Source: CAD feature listing. Evaluate the final solid. Frame: model axes, mm. Face numbers are marked on the shaded views. Give positions to 0.01 mm unless a question says otherwise; leave off trailing zeros. Order: outer loops, then holes, each group sorted by start corner. A loop starts at its lowest first (then second) coordinate and runs counter-clockwise, first axis right, second up. Notation, with made-up numbers: (-37, -14.5) -> (7, -14.5) arc R31 cw to (7, 10.5) -> close; hole circle Ø3 at (81.25, 16). An arc over 180 degrees is marked (long way). Answer in a Markdown table with one row per item.
Autodesk Inventor part; units mm, degrees
ref_plane "mss_or_XY" through (0, 0, 0) normal (1, 0, 0) x (0, 0, -1)
ref_plane "mss_or_YZ" through (0, 0, 0) normal (0, 0, -1) x (0, 1, 0)
ref_plane "mss_or_ZX" through (0, 0, 0) normal (0, 1, 0) x (1, 0, 0)
sketch "Sketch_2" plane through (0, 0, 0) normal (0, 0, 1) x (1, 0, 0)
  line L0 (2.5, 0) -> (0, 0)
  line L1 (0, 2.92) -> (0, 2.52)
  line L2 (0, 2.52) -> (0.8975, 2.52)
  arc A0 (1.6025, 2.52) -> (0.8975, 2.52) centre (1.25, 2.25) ccw
  line L3 (1.6025, 2.52) -> (2.4438, 2.52)
  line L4 (2.4438, 2.52) -> (2.4438, 2.616)
  line L5 (2.4438, 2.616) -> (2.5, 2.616)
  line L6 (2.5, 2.616) -> (2.5, 2.92)
  arc A1 (2.5, 2.92) -> (2.42, 3) centre (2.42, 2.92) ccw
  line L7 (2.42, 3) -> (0.08, 3)
  arc A2 (0.08, 3) -> (0, 2.92) centre (0.08, 2.92) ccw
revolve "Revolution1" add sketch "Sketch_2" angle 360 about axis through (2.5, 0, 0) along (1, 0, 0)
ref_plane "mss_or_XY" through (0, 0, 0) normal (1, 0, 0) x (0, 0, -1)
ref_plane "mss_or_YZ" through (0, 0, 0) normal (0, 0, -1) x (0, 1, 0)
ref_plane "mss_or_ZX" through (0, 0, 0) normal (0, 1, 0) x (1, 0, 0)
ref_plane "mss_or11_XY" through (2.5, 0, 0) normal (1, 0, 0) x (0, 0, -1)
ref_plane "mss_or11_YZ" through (2.5, 0, 0) normal (0, 0, -1) x (0, 1, 0)
ref_plane "mss_or11_ZX" through (2.5, 0, 0) normal (0, 1, 0) x (1, 0, 0)
ref_plane "mss_or2_1_XY" through (1, 2.25, 0) normal (1, 0, 0) x (0, 0, -1)
ref_plane "mss_or2_1_YZ" through (1, 2.25, 0) normal (0, 0, -1) x (0, 1, 0)
ref_plane "mss_or2_1_ZX" through (1, 2.25, 0) normal (0, 1, 0) x (1, 0, 0)
ref_plane "mss_or2_2_XY" through (1, 1.7236, 1.4463) normal (1, 0, 0) x (0, 0, -1)
ref_plane "mss_or2_2_YZ" through (1, 1.7236, 1.4463) normal (0, 0, -1) x (0, 1, 0)
ref_plane "mss_or2_2_ZX" through (1, 1.7236, 1.4463) normal (0, 1, 0) x (1, 0, 0)
ref_plane "mss_or2_3_XY" through (1, 0.3907, 2.2158) normal (1, 0, 0) x (0, 0, -1)
ref_plane "mss_or2_3_YZ" through (1, 0.3907, 2.2158) normal (0, 0, -1) x (0, 1, 0)
ref_plane "mss_or2_3_ZX" through (1, 0.3907, 2.2158) normal (0, 1, 0) x (1, 0, 0)
ref_plane "mss_or2_4_XY" through (1, -1.125, 1.9486) normal (1, 0, 0) x (0, 0, -1)
ref_plane "mss_or2_4_YZ" through (1, -1.125, 1.9486) normal (0, 0, -1) x (0, 1, 0)
ref_plane "mss_or2_4_ZX" through (1, -1.125, 1.9486) normal (0, 1, 0) x (1, 0, 0)
ref_plane "mss_or2_5_XY" through (1, -2.1143, 0.7695) normal (1, 0, 0) x (0, 0, -1)
ref_plane "mss_or2_5_YZ" through (1, -2.1143, 0.7695) normal (0, 0, -1) x (0, 1, 0)
ref_plane "mss_or2_5_ZX" through (1, -2.1143, 0.7695) normal (0, 1, 0) x (1, 0, 0)
ref_plane "mss_or2_6_XY" through (1, -2.1143, -0.7695) normal (1, 0, 0) x (0, 0, -1)
ref_plane "mss_or2_6_YZ" through (1, -2.1143, -0.7695) normal (0, 0, -1) x (0, 1, 0)
ref_plane "mss_or2_6_ZX" through (1, -2.1143, -0.7695) normal (0, 1, 0) x (1, 0, 0)
ref_plane "mss_or2_7_XY" through (1, -1.125, -1.9486) normal (1, 0, 0) x (0, 0, -1)
ref_plane "mss_or2_7_YZ" through (1, -1.125, -1.9486) normal (0, 0, -1) x (0, 1, 0)
ref_plane "mss_or2_7_ZX" through (1, -1.125, -1.9486) normal (0, 1, 0) x (1, 0, 0)
ref_plane "mss_or2_8_XY" through (1, 0.3907, -2.2158) normal (1, 0, 0) x (0, 0, -1)
ref_plane "mss_or2_8_YZ" through (1, 0.3907, -2.2158) normal (0, 0, -1) x (0, 1, 0)
ref_plane "mss_or2_8_ZX" through (1, 0.3907, -2.2158) normal (0, 1, 0) x (1, 0, 0)
ref_plane "mss_or2_9_XY" through (1, 1.7236, -1.4463) normal (1, 0, 0) x (0, 0, -1)
ref_plane "mss_or2_9_YZ" through (1, 1.7236, -1.4463) normal (0, 0, -1) x (0, 1, 0)
ref_plane "mss_or2_9_ZX" through (1, 1.7236, -1.4463) normal (0, 1, 0) x (1, 0, 0)
ref_plane "mss_or21_1_XY" through (1.25, 2.25, 0) normal (1, 0, 0) x (0, 0, -1)
ref_plane "mss_or21_1_YZ" through (1.25, 2.25, 0) normal (0, 0, -1) x (0, 1, 0)
ref_plane "mss_or21_1_ZX" through (1.25, 2.25, 0) normal (0, 1, 0) x (1, 0, 0)
ref_plane "mss_or21_2_XY" through (1.25, 1.7236, 1.4463) normal (1, 0, 0) x (0, 0, -1)
ref_plane "mss_or21_2_YZ" through (1.25, 1.7236, 1.4463) normal (0, 0, -1) x (0, 1, 0)
ref_plane "mss_or21_2_ZX" through (1.25, 1.7236, 1.4463) normal (0, 1, 0) x (1, 0, 0)
ref_plane "mss_or21_3_XY" through (1.25, 0.3907, 2.2158) normal (1, 0, 0) x (0, 0, -1)
ref_plane "mss_or21_3_YZ" through (1.25, 0.3907, 2.2158) normal (0, 0, -1) x (0, 1, 0)
ref_plane "mss_or21_3_ZX" through (1.25, 0.3907, 2.2158) normal (0, 1, 0) x (1, 0, 0)
ref_plane "mss_or21_4_XY" through (1.25, -1.125, 1.9486) normal (1, 0, 0) x (0, 0, -1)
ref_plane "mss_or21_4_YZ" through (1.25, -1.125, 1.9486) normal (0, 0, -1) x (0, 1, 0)
ref_plane "mss_or21_4_ZX" through (1.25, -1.125, 1.9486) normal (0, 1, 0) x (1, 0, 0)
ref_plane "mss_or21_5_XY" through (1.25, -2.1143, 0.7695) normal (1, 0, 0) x (0, 0, -1)
ref_plane "mss_or21_5_YZ" through (1.25, -2.1143, 0.7695) normal (0, 0, -1) x (0, 1, 0)
ref_plane "mss_or21_5_ZX" through (1.25, -2.1143, 0.7695) normal (0, 1, 0) x (1, 0, 0)
ref_plane "mss_or21_6_XY" through (1.25, -2.1143, -0.7695) normal (1, 0, 0) x (0, 0, -1)
ref_plane "mss_or21_6_YZ" through (1.25, -2.1143, -0.7695) normal (0, 0, -1) x (0, 1, 0)
ref_plane "mss_or21_6_ZX" through (1.25, -2.1143, -0.7695) normal (0, 1, 0) x (1, 0, 0)
ref_plane "mss_or21_7_XY" through (1.25, -1.125, -1.9486) normal (1, 0, 0) x (0, 0, -1)
ref_plane "mss_or21_7_YZ" through (1.25, -1.125, -1.9486) normal (0, 0, -1) x (0, 1, 0)
ref_plane "mss_or21_7_ZX" through (1.25, -1.125, -1.9486) normal (0, 1, 0) x (1, 0, 0)
ref_plane "mss_or21_8_XY" through (1.25, 0.3907, -2.2158) normal (1, 0, 0) x (0, 0, -1)
ref_plane "mss_or21_8_YZ" through (1.25, 0.3907, -2.2158) normal (0, 0, -1) x (0, 1, 0)
ref_plane "mss_or21_8_ZX" through (1.25, 0.3907, -2.2158) normal (0, 1, 0) x (1, 0, 0)
ref_plane "mss_or21_9_XY" through (1.25, 1.7236, -1.4463) normal (1, 0, 0) x (0, 0, -1)
ref_plane "mss_or21_9_YZ" through (1.25, 1.7236, -1.4463) normal (0, 0, -1) x (0, 1, 0)
ref_plane "mss_or21_9_ZX" through (1.25, 1.7236, -1.4463) normal (0, 1, 0) x (1, 0, 0)
properties part number "WA673SA Outer ring"
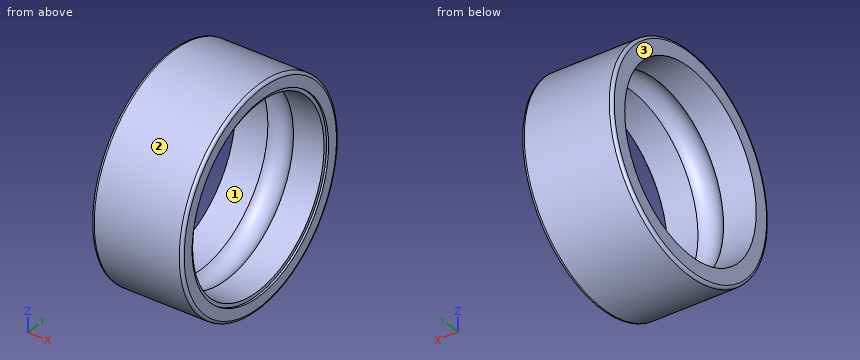
(1) First-contact query: pin 1 Ø3 at (y, z) = (0, 0) entering from +X. Flat tip, straight axial feed; report the tip coordinate or a pass-through.
A:
| item | result |
|---|---|
| pin 1 | passes through |
(2) Pull-direction query (Z, two-part tool) for the marked faces 1, 2 and 3; classes: +Z half, -Z half, draft (parallel to the pull), parting line (faces both ways), or undercut.
A:
| item | result |
|---|---|
| face 1 | undercut |
| face 2 | parting line |
| face 3 | draft |
(3) Section query A-A (z = 0). Return the cut outline in (x, y), plus the area to 3 significant figures.
A:
| item | result |
|---|---|
| outline | (0, -2.92) arc R0.08 ccw to (0.08, -3) -> (2.42, -3) arc R0.08 ccw to (2.5, -2.92) -> (2.5, -2.62) -> (2.44, -2.62) -> (2.44, -2.52) -> (1.6, -2.52) arc R0.44 cw to (0.9, -2.52) -> (0, -2.52) -> close; (0, 2.52) -> (0.9, 2.52) arc R0.44 cw to (1.6, 2.52) -> (2.44, 2.52) -> (2.44, 2.62) -> (2.5, 2.62) -> (2.5, 2.92) arc R0.08 ccw to (2.42, 3) -> (0.08, 3) arc R0.08 ccw to (0, 2.92) -> close |
| area | 2.21 mm^2 |
(4) Ray query, probe 1 along Z at (x, y) = (2.05, 0); probe 2 along X at (y, z) = (-2.5, 0.55); probe 3 along Z at (x, y) = (1.35, 0.25). Return the intervals inside material, ascending.
A:
| item | result |
|---|---|
| probe 1 | z = -3 to -2.52, 2.52 to 3 |
| probe 2 | x = 0 to 0.93, 1.57 to 2.44 |
| probe 3 | z = -2.99 to -2.67, 2.67 to 2.99 |
(5) Section query C-C (x = 0.3). Return the cut outline in (y, z).
A:
| item | result |
|---|---|
| outline | circle Ø6 at (0, 0); hole circle Ø5.04 at (0, 0) |
